Part model, mm, in its own coordinate system. A direction names the side the tool comes from. Coordinates: 2 decimals unless noted, no trailing zeros. Loops run counter-clockwise (first coordinate to the right, second up) from the corner with the lowest first, then second, coordinate; pieces in that order, holes last. Notation, with made-up numbers: (-21.75, 10) - (24.25, 10) arc R24 cw to (24.25, 27) - close; hole circle Ø3 at (-26, 63.5). An arc over 180 degrees is marked (long way). Use a Markdown table: item, result. Add a question column.
1. Pull direction X, two halves, no side cores. Call faces 3 (the flat face through (0, 20, 6)), 4 (the flat face through (0, 30, 0)), 5 (the cylindrical face through (1.302, 14.79, 9.915)): pulls with the +X half, pulls with the -X half, needs draft (parallel to the pull), parting line crosses it, or undercut.
2. Wall check: probe 1 along Y at (x, z) = (0, -2.75); probe 2 along Y at (x, z) = (-2.25, 11.5); probe 3 along Y at (x, z) = (-1.5, -5). Give the ranges that are in metal, low to high. Write a range as [from, to].
3. 3-axis set-ups, long thin cutter, end or side, ignore diameter. For faces 1 (the flat face through (3, 0, -10)), 2 (the flat face through (0, -4, 0)): which of +Z, -Z, +X, -X, +Y, -Y reach the whole face in a straight line?
4. Drop flat-ended pins along their axis: pin 1 (6.5 mm diameter, centred on x = 0, y = 19.83, fed in from -Z); pin 2 (1 mm diameter, centred on x = -0.5, y = 25.5, fed in from -Z); pin 3 (2 mm diameter, centred on x = -5.5, y = 3.5, fed in from +Z). Give the stop position or say it passes through.
5. Band-saw the part on C-C, the plane y = 13.5. Give the cut face in (x, z), plus the area to 3 significant figures.
6. Band-saw the part on B-B, the plane x = 0. Give the cut face in (y, z).
7. Band-saw the part on A-A, the plane z = 5.5. Give the cut face in (x, y), plus the area to 3 significant figures.
8. Band-saw the part on D-D, the plane z = 12. Give the cut face in (x, y), plus the area to 3 significant figures.
from build123d import *

# Parameters (mm, degrees)
F0_R     = 15
F1_DEPTH = 4
F2_R     = 10
F3_DEPTH = 30
F4_R     = 4
F5_DEPTH = 27
F6_DEPTH = 6


with BuildPart() as f1:
    # F0 (on Front) → F1 (new body)
    with BuildSketch(Plane.XZ):
        Circle(F0_R)
    extrude(amount=F1_DEPTH)

    # F2 (on face) → F3 (join)
    with BuildSketch(Plane(origin=(0, 0, 0), x_dir=(-1, 0, 0), z_dir=(0, 1, 0))):
        Circle(F2_R)
    extrude(amount=F3_DEPTH)

    # F4 (on Top) → F5 (cut)
    with BuildSketch(Plane.XY):
        with Locations((0, 19.828215)):
            Circle(F4_R)
    extrude(amount=-F5_DEPTH, mode=Mode.SUBTRACT)

    # F4 (on Top) → F6 (cut)
    with BuildSketch(Plane.XY):
        with Locations((0, 19.828215)):
            Circle(F4_R)
    extrude(amount=F6_DEPTH, mode=Mode.SUBTRACT)


solid = f1.part
Geometry check:
| question | item | result |
|---|---|---|
| 1 | face 3 | undercut |
| 1 | face 4 | needs draft |
| 1 | face 5 | parting line crosses it |
| 2 | probe 1 | y = [-4, 15.83], [23.83, 30] |
| 2 | probe 2 | y = [-4, 0] |
| 2 | probe 3 | y = [-4, 16.12], [23.54, 30] |
| 3 | face 1 | +Y |
| 3 | face 2 | +Z, -Z, +X, -X, -Y |
| 4 | pin 1 | stops at z = 6 |
| 4 | pin 2 | stops at z = -10 |
| 4 | pin 3 | stops at z = 8.93 |
| 5 | outline | circle Ø20 at (0, 0) |
| 5 | area | 314 mm^2 |
| 6 | outline | (-4, -15) - (0, -15) - (0, -10) - (15.83, -10) - (15.83, 6) - (23.83, 6) - (23.83, -10) - (30, -10) - (30, 10) - (0, 10) - (0, 15) - (-4, 15) - close |
| 7 | outline | (-13.96, -4) - (13.96, -4) - (13.96, 0) - (8.35, 0) - (8.35, 30) - (-8.35, 30) - (-8.35, 0) - (-13.96, 0) - close; hole circle Ø8 at (0, 19.83) |
| 7 | area | 562 mm^2 |
| 8 | outline | (-9, -4) - (9, -4) - (9, 0) - (-9, 0) - close |
| 8 | area | 72.0 mm^2 |
